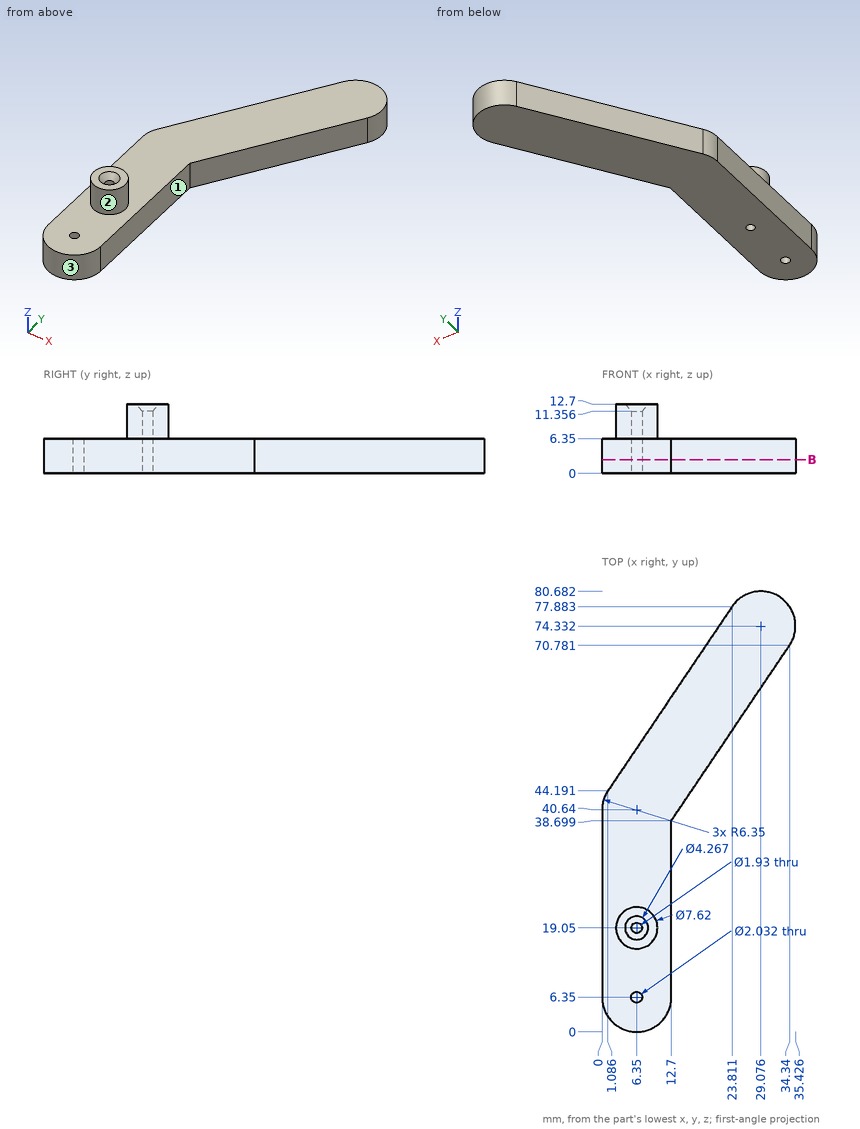
Source: three-view drawing plus pictorial views. Frame: mm from the lowest corner of the part. A direction names the side the tool comes from. Round coordinates to 2 decimals unless told otherwise and drop trailing zeros. Answer in a Markdown table with one row per item.
Item 1: Section query B-B (z = 2.5). Give the number of separate pieces and of enclosed holes in the cut face, then the cut area to 3 significant figures.
Model answer:
| item | result |
|---|---|
| separate pieces | 1 |
| enclosed holes | 2 |
| area | 1,070 mm² |
Item 2: Reachability of the marked faces 1, 2 and 3 from +Z, -Z, +X, -X, +Y, -Y: full face, straight path, thin tool, end or side. Return the list, or none.
Model answer:
| item | result |
|---|---|
| face 1 | +Z, -Z, +X, -Y |
| face 2 | +Z |
| face 3 | +Z, -Z, -Y |
Item 3: Line query: line 1 (Y direction, x = 6.35, z = 4.25) (1 decimal); line 2 (Z direction, x = 7.5, y = 40); line 3 (X direction, y = 19.05, z = 3) (1 decimal). Output: solid intervals per line, ascending.
Model answer:
| item | result |
|---|---|
| line 1 | y = 0 to 5.3, 7.4 to 18.1, 20 to 52 |
| line 2 | z = 0 to 6.35 |
| line 3 | x = 0 to 5.4, 7.3 to 12.7 |
Item 4: Pin query (flat end, axial travel): pin 1 (3 mm diameter, centred on x = 4, z = 10, fed in from -Y); pin 2 (1.5 mm diameter, centred on y = 52, z = 3.5, fed in from +X); pin 3 (6 mm diameter, centred on x = 13, y = 56, fed in from +Z). Return the tip coordinate at first contact, or that it passes through.
Model answer:
| item | result |
|---|---|
| pin 1 | stops at y = 15.34 |
| pin 2 | stops at x = 22.18 |
| pin 3 | stops at z = 6.35 |
